from build123d import *

# Parameters (mm, degrees)
EXTRUDE_1_DEPTH     = 6
FILLET_1_R          = 2
FILLET_2_R          = 2
FILLET_3_R          = 0.3
SKETCH_2_R          = 2
CUT_EXTRUDE_1_DEPTH = 6


with BuildPart() as part:
    # 草图1 → 凸台-拉伸1 (new body)
    with BuildSketch(Plane.XY):
        Polygon((-3, 4.3), (3, 4.3), (3, 3.3), (5.1, 3.3), (5.1, 2.3), (2.8, 0), (-2.8, 0), (-5.1, 2.3), (-5.1, 3.3), (-3, 3.3), align=None)
    extrude(amount=EXTRUDE_1_DEPTH)

    # 圆角1
    fillet_1_edges = [part.edges().sort_by_distance(p)[0] for p in [
        (-3, 3.8, 0),
        (3, 3.8, 6),
    ]]
    fillet(fillet_1_edges, radius=FILLET_1_R)

    # 圆角2
    fillet_2_edges = [part.edges().sort_by_distance(p)[0] for p in [
        (-5.1, 2.8, 0),
        (5.1, 2.8, 6),
    ]]
    fillet(fillet_2_edges, radius=FILLET_2_R)

    # 圆角3
    fillet_3_edges = [part.edges().sort_by_distance(p)[0] for p in [
        (-3, 3.8, 6),
        (3, 3.8, 0),
        (-5.1, 2.8, 6),
        (5.1, 2.8, 0),
    ]]
    fillet(fillet_3_edges, radius=FILLET_3_R)

    # 草图2 → 切除-拉伸1 (cut)
    with BuildSketch(Plane(origin=(0, 4.3, 0), x_dir=(1, 0, 0), z_dir=(0, 1, 0))):
        with Locations((0, -3)):
            Circle(SKETCH_2_R)
    extrude(amount=-CUT_EXTRUDE_1_DEPTH, mode=Mode.SUBTRACT)


solid = part.part
Part model, mm, in its own coordinate system. A direction names the side the tool comes from. Coordinates: 2 decimals unless noted, no trailing zeros. Loops run counter-clockwise (first coordinate to the right, second up) from the corner with the lowest first, then second, coordinate; pieces in that order, holes last. Notation, with made-up numbers: (21.5, 23.25) -> (58.5, 23.25) arc R17 ccw to (58.5, 39.25) -> close; hole circle Ø11 at (69.5, 50). An arc over 180 degrees is marked (long way). Use a Markdown table: item, result. Add a question column.
Item 1: Probe probe 1 along Z at (x, y) = (0, 3.05); probe 2 along X at (y, z) = (3.2, 3); probe 3 along X at (y, z) = (1.55, 3). List the from-to ranges inside material, lowest first.
Item 2: Band-saw the part on C-C on y = 2.45. Write the cut outline in (x, z).
Item 3: Band-saw the part on B-B on x = 0. Write the cut outline in (y, z), plus the area to 3 significant figures.
Item 4: Band-saw the part on A-A on z = 3. Write the cut outline in (x, y), plus the area to 3 significant figures.
Item 5: Flat gauge pins, fed straight in: P1, Ø2.5, axis at x = 0, z = 3, coming from the +Y side; P2, Ø1.5, axis at y = 0.5, z = 2, coming from the -X side. Where does each tip first touch, or does it go through?
Item 6: Band-saw the part on D-D on x = -1.75. Write the cut outline in (y, z), plus the area to 3 significant figures.
Item 7: Which spindle directions (+Z, -Z, +X, -X, +Y, -Y) get a long thin tool onto all of the face, cutting with end or side? Do faces 1 (the cylindrical face through (-2.43, 3.81, 0.6)), 2 (the flat face through (-3, 4, 4)), 3 (the cylindrical face through (2.43, 3.79, 5.4)). Say none if no direction does.
Item 8: Pull direction Z, two halves, no side cores. Call faces 4 (the cylindrical face through (0, 2, 5)), 5 (the cylindrical face through (4.3, 2.4, 5.6)), 6 (the flat face through (-3.9, 1.1, 3)): +Z half, -Z half, draft (parallel to the pull), parting line (faces both ways), or undercut.
Geometry says:
| question | item | result |
|---|---|---|
| 1 | probe 1 | 0 to 1, 5 to 6 |
| 1 | probe 2 | -5.1 to -2, 2 to 5.1 |
| 1 | probe 3 | -4.35 to -2, 2 to 4.35 |
| 2 | outline | (-5.1, 2) arc R2 ccw to (-3.1, 0) -> (4.8, 0) arc R0.3 ccw to (5.1, 0.3) -> (5.1, 4) arc R2 ccw to (3.1, 6) -> (-4.8, 6) arc R0.3 ccw to (-5.1, 5.7) -> close; hole circle Ø4 at (0, 3) |
| 3 | outline | (0, 0) -> (4.3, 0) -> (4.3, 1) -> (0, 1) -> close; (0, 5) -> (4.3, 5) -> (4.3, 6) -> (0, 6) -> close |
| 3 | area | 8.60 mm² |
| 4 | outline | (-5.1, 2.3) -> (-2.8, 0) -> (-2, 0) -> (-2, 4.3) -> (-3, 4.3) -> (-3, 3.3) -> (-5.1, 3.3) -> close; (2, 0) -> (2.8, 0) -> (5.1, 2.3) -> (5.1, 3.3) -> (3, 3.3) -> (3, 4.3) -> (2, 4.3) -> close |
| 4 | area | 17.2 mm² |
| 5 | P1 | through |
| 5 | P2 | x = -4.05 |
| 6 | outline | (0, 0) -> (3.3, 0) -> (3.3, 0.15) -> (4.3, 0.15) -> (4.3, 2.03) -> (0, 2.03) -> close; (0, 3.97) -> (4.3, 3.97) -> (4.3, 6) -> (0, 6) -> close |
| 6 | area | 17.3 mm² |
| 7 | face 1 | -Z, -X, +Y |
| 7 | face 2 | +Z, -Z, -X, +Y |
| 7 | face 3 | +Z, +X, +Y |
| 8 | face 4 | undercut |
| 8 | face 5 | +Z half |
| 8 | face 6 | draft |
